from build123d import *

# Parameters (mm, degrees)
SKETCH1_W           = 498.348
SKETCH1_H           = 145.542
BOSS_EXTRUDE1_DEPTH = 1.143
SKETCH2_W           = 69.85
SKETCH2_H           = 2.286
BOSS_EXTRUDE2_DEPTH = 3.175
LPATTERN1_COUNT     = 5
LPATTERN1_PITCH     = 98.8568
SKETCH3_W           = 3.175
SKETCH3_H           = 38.1
CUT_EXTRUDE1_DEPTH  = 3.286
SKETCH5_W           = 2.286
SKETCH5_H           = 72.771
CUT_EXTRUDE2_DEPTH  = 3.286
LPATTERN2_COUNT     = 4
LPATTERN2_PITCH     = 98.8568


with BuildPart() as part:
    # Sketch1 → Boss-Extrude1 (new body, symmetric)
    with BuildSketch(Plane(origin=(0, 0, 0), x_dir=(1, 0, 0), z_dir=(0, 1, 0))):
        Rectangle(SKETCH1_W, SKETCH1_H)
    extrude(amount=BOSS_EXTRUDE1_DEPTH, both=True)

    # Sketch2 → Boss-Extrude2 (add)
    with BuildSketch(Plane(origin=(0, 0, -72.771), x_dir=(-1, 0, 0), z_dir=(0, 0, -1))):
        with Locations((-197.7136, 0)):
            Rectangle(SKETCH2_W, SKETCH2_H)
    boss_extrude2 = extrude(amount=BOSS_EXTRUDE2_DEPTH)

    # LPattern1: Boss-Extrude2 ×5
    with Locations(*[(-i * LPATTERN1_PITCH, 0, 0) for i in range(1, LPATTERN1_COUNT)]):
        add(boss_extrude2)

    # Sketch3 → Cut-Extrude1 (cut, through all)
    with BuildSketch(Plane.XZ.offset(1.143)):
        with Locations((-247.5865, 53.721)):
            Rectangle(SKETCH3_W, SKETCH3_H)
    cut_extrude1 = extrude(amount=-CUT_EXTRUDE1_DEPTH, mode=Mode.SUBTRACT)

    # Mirror2: Cut-Extrude1 across plane
    add(cut_extrude1.mirror(Plane(origin=(0, 0, 0), x_dir=(0, 0, 1), z_dir=(1, 0, 0))), mode=Mode.SUBTRACT)

    # Sketch5 → Cut-Extrude2 (cut, through all)
    with BuildSketch(Plane.XZ.offset(1.143)):
        with Locations((-148.2852, 36.3855)):
            Rectangle(SKETCH5_W, SKETCH5_H)
    cut_extrude2 = extrude(amount=-CUT_EXTRUDE2_DEPTH, mode=Mode.SUBTRACT)

    # LPattern2: Cut-Extrude2 ×4
    with Locations(*[(i * LPATTERN2_PITCH, 0, 0) for i in range(1, LPATTERN2_COUNT)]):
        add(cut_extrude2, mode=Mode.SUBTRACT)


solid = part.part
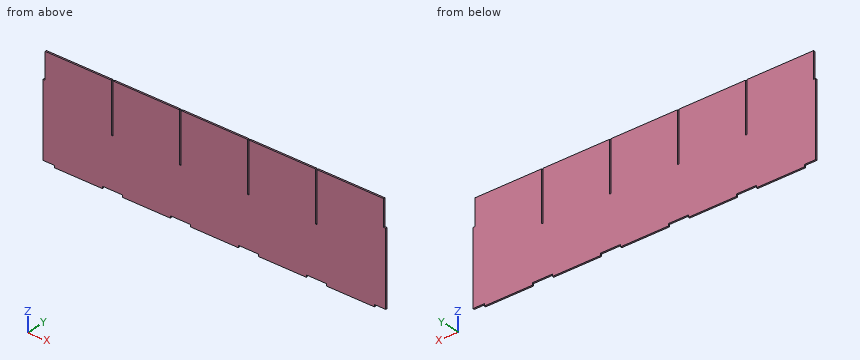
Here's how the part is built. I have some questions about the finished solid (model axes, mm). Give positions to 0.01 mm unless a question says otherwise; leave off trailing zeros. Order: outer loops, then holes, each group sorted by start corner. A loop starts at its lowest first (then second) coordinate and runs counter-clockwise, first axis right, second up. Notation, with made-up numbers: (15, 76.25) -> (63, 76.25) arc R4 ccw to (63, 82.25) -> close; hole circle Ø4 at (22.25, 25). An arc over 180 degrees is marked (long way). Use a Markdown table: item, result. Add a question column.
Item 1: Imagine slicing it at B-B on z = 13. Please give me the cut outline in (x, y).
Item 2: Will these pins go through, and if not, where does the flat tip stop? pin 1 (1.1 mm diameter, centred on y = 0, z = 46.5, fed in from +X); pin 2 (1.1 mm diameter, centred on y = 0.5, z = -74, fed in from -X); pin 3 (1.1 mm diameter, centred on x = -148.5, y = -0.5, fed in from +Z).
Item 3: I need wall thicknesses on line 1 (X direction, y = -0.7, z = 57); line 2 (X direction, y = -0.05, z = 20.5); line 3 (Z direction, x = -55, y = 0.4). Which ranges of each line are inside material? Lowest first, please.
Item 4: Imagine slicing it at A-A on z = 60. Please give me the cut outline in (x, y).
Data:
| question | item | result |
|---|---|---|
| 1 | outline | (-249.17, -1.14) -> (-149.43, -1.14) -> (-149.43, 1.14) -> (-249.17, 1.14) -> close; (-147.14, -1.14) -> (-50.57, -1.14) -> (-50.57, 1.14) -> (-147.14, 1.14) -> close; (-48.29, -1.14) -> (48.29, -1.14) -> (48.29, 1.14) -> (-48.29, 1.14) -> close; (50.57, -1.14) -> (147.14, -1.14) -> (147.14, 1.14) -> (50.57, 1.14) -> close; (149.43, -1.14) -> (249.17, -1.14) -> (249.17, 1.14) -> (149.43, 1.14) -> close |
| 2 | pin 1 | stops at x = 246 |
| 2 | pin 2 | stops at x = -232.64 |
| 2 | pin 3 | stops at z = 0 |
| 3 | line 1 | x = -246 to -149.43, -147.14 to -50.57, -48.29 to 48.29, 50.57 to 147.14, 149.43 to 246 |
| 3 | line 2 | x = -249.17 to -149.43, -147.14 to -50.57, -48.29 to 48.29, 50.57 to 147.14, 149.43 to 249.17 |
| 3 | line 3 | z = -72.77 to 72.77 |
| 4 | outline | (-246, -1.14) -> (-149.43, -1.14) -> (-149.43, 1.14) -> (-246, 1.14) -> close; (-147.14, -1.14) -> (-50.57, -1.14) -> (-50.57, 1.14) -> (-147.14, 1.14) -> close; (-48.29, -1.14) -> (48.29, -1.14) -> (48.29, 1.14) -> (-48.29, 1.14) -> close; (50.57, -1.14) -> (147.14, -1.14) -> (147.14, 1.14) -> (50.57, 1.14) -> close; (149.43, -1.14) -> (246, -1.14) -> (246, 1.14) -> (149.43, 1.14) -> close |
